from build123d import *
from build123d.topology import SkipClean

# Parameters (mm, degrees)
SKETCH1_R               = 5
BOSS_EXTRUDE1_DEPTH     = 50
CUT_EXTRUDE1_START      = 4
SKETCH1_3_R             = 4
CUT_EXTRUDE1_DEPTH      = 50
BOSS_EXTRUDE2_START     = 10
BOSS_EXTRUDE2_DEPTH     = 10
FILLET3_R               = 4
CUT_EXTRUDE2_DEPTH      = 51.806003597
CUT_EXTRUDE2_DEPTH_BACK = 51.806003597
SKETCH3_R               = 2.5


with BuildPart() as part:
    # Sketch1 → Boss-Extrude1 (new body)
    with BuildSketch(Plane(origin=(0, 0, 0), x_dir=(1, 0, 0), z_dir=(0, 1, 0))):
        with Locations(Location((0, 0, 0), (0, 0, 270))):
            Circle(SKETCH1_R)
    extrude(amount=BOSS_EXTRUDE1_DEPTH)

    # Sketch1<3> → Cut-Extrude1 (cut)
    with BuildSketch(Plane(origin=(0, 0, 0), x_dir=(1, 0, 0), z_dir=(0, 1, 0)).offset(CUT_EXTRUDE1_START)):
        with Locations(Location((0, 0, 0), (0, 0, 270))):
            Circle(SKETCH1_3_R)
    extrude(amount=CUT_EXTRUDE1_DEPTH, mode=Mode.SUBTRACT)

    # Sketch2 → Boss-Extrude2 (add)
    with SkipClean():  # the faces are left unmerged after this step: merging them gives an invalid solid
        with BuildSketch(Plane.XZ.offset(BOSS_EXTRUDE2_START)):
            with BuildLine():
                Line((-2.5, 4.330127019), (-2.5, -4.330127019))
                ThreePointArc((-2.5, -4.330127019), (-5, 0), (-2.5, 4.330127019))
            make_face()
            with BuildLine():
                Line((2.5, 4.330127019), (2.5, -4.330127019))
                ThreePointArc((2.5, -4.330127019), (5, 0), (2.5, 4.330127019))
            make_face()
        extrude(amount=-BOSS_EXTRUDE2_DEPTH)

    # Fillet3
    # the kernel refuses this fillet: 4 mm, written as the material it takes off along each edge
    with BuildSketch(Plane(origin=(0, -10, 0), x_dir=(0.9956817269656716, 0, -0.09283263750781805), z_dir=(0.09283263750781805, 0, 0.9956817269656716))) as fillet3_piece_1:
        with BuildLine():
            CenterArc((5 - FILLET3_R, FILLET3_R), FILLET3_R, 270, 90)
            Line((5 - FILLET3_R, 0), (5, 0))
            Line((5, 0), (5, FILLET3_R))
        make_face()
    revolve(axis=Axis((0, -10, 0), (0, 1, 0)), revolution_arc=349.34682448, mode=Mode.SUBTRACT)
    with BuildSketch(Plane(origin=(0, -10, 0), x_dir=(-0.9956817269656714, 0, -0.09283263750781937), z_dir=(-0.09283263750781937, 0, 0.9956817269656714))) as fillet3_piece_2:
        with BuildLine():
            CenterArc((5 - FILLET3_R, -FILLET3_R), FILLET3_R, 0, 90)
            Line((5 - FILLET3_R, 0), (5, 0))
            Line((5, 0), (5, -FILLET3_R))
        make_face()
    revolve(axis=Axis((0, -10, 0), (0, -1, 0)), revolution_arc=349.34682448, mode=Mode.SUBTRACT)

    # Sketch3 → Cut-Extrude2 (cut, two sides: drawn at the far end of the back side and taken through both)
    with BuildSketch(Plane(origin=(-2.5, 0, 0), x_dir=(0, 0, -1), z_dir=(1, 0, 0)).offset(-CUT_EXTRUDE2_DEPTH_BACK)):
        with Locations((0, -6)):
            Circle(SKETCH3_R)
    extrude(amount=CUT_EXTRUDE2_DEPTH + CUT_EXTRUDE2_DEPTH_BACK, mode=Mode.SUBTRACT)


solid = part.part
Input: part model. Units: mm. Frame: model coordinates. A direction names the side the tool comes from. Give positions to 0.01 mm unless a question says otherwise; leave off trailing zeros. Order: outer loops, then holes, each group sorted by start corner. A loop starts at its lowest first (then second) coordinate and runs counter-clockwise, first axis right, second up. Notation, with made-up numbers: M 63.25,-10.75 L 117.25,-10.75 A18 cw 117.25,2.25 Z; hole C 37,56.25 d6. An arc over 180 degrees is marked long. Answer as a JSON object with one key per item and string values.
1. Ray query, line 1 (Z direction, x = 0, y = 41); line 2 (X direction, y = -5, z = -2.5). Return the intervals inside material, ascending. Write a range as [from, to].
Result sheet:
{"line 1": "[-5, -4], [4, 5]", "line 2": "[-4.33, -2.5], [2.5, 4.33]"}
2. First-contact query: P1, Ø3, axis at x = -4, y = 26, coming from the -Z side; P2, Ø4, axis at x = -1, z = -1.5, coming from the +Y side; P3, Ø4, axis at y = -6, z = 0, coming from the +X side; P4, Ø1, axis at x = 1.5, z = -4, coming from the -Y side. Flat tips, straight axial feed; report the tip coordinate or a pass-through.
Result sheet:
{"P1": "z = -4.33", "P2": "y = 4", "P3": "through", "P4": "y = 0"}
3. Reachability of faces 4 (the flat face through (0, 4, 0)), 5 (the flat face through (-2.5, -3, 0)) from +Z, -Z, +X, -X, +Y, -Y: full face, straight path, thin tool, end or side. Return the list, or none.
Result sheet:
{"face 4": "+Y", "face 5": "+Z, -Z, -Y"}
4. Cut plane B-B, the plane y = 2.5. Output: boundary loops of the cut face in (x, z).
Result sheet:
{"outline": "C 0,0 d10"}
5. Cut plane C-C, the plane z = 1.5. State how many separate pieces and enclosed holes the cut face has, and give its area (3 significant figures).
Result sheet:
{"separate pieces": "3", "enclosed holes": "0", "area": "157 mm²"}
6. Cut plane A-A, the plane x = 0. Output: boundary loops of the cut face in (y, z).
Result sheet:
{"outline": "M 0,-5 L 50,-5 L 50,-4 L 4,-4 L 4,4 L 50,4 L 50,5 L 0,5 Z"}
7. Pull-direction query (Z, two-part tool) for faces 1 (the cylindrical face through (-3.49, -3.52, 0.33)), 2 (the flat face through (0, 0, 0)), 3 (the cylindrical face through (3.46, -3.52, 0.33)); classes: +Z half, -Z half, draft (parallel to the pull), parting line (faces both ways), or undercut.
Result sheet:
{"face 1": "undercut", "face 2": "draft", "face 3": "undercut"}
